Could you check a few things on this model? Use its own coordinates, in mm. A direction names the side the tool comes from. Round coordinates to 2 decimals unless told otherwise and drop trailing zeros. Loops run counter-clockwise (first coordinate to the right, second up) from the corner with the lowest first, then second, coordinate; pieces in that order, holes last. Notation, with made-up numbers: M 50.25,48 L 102.25,48 A21 ccw 102.25,66 Z; hole C 47.25,84 d10. An arc over 180 degrees is marked long. Answer in a Markdown table with one row per item.
```python
from build123d import *

# Parameters (mm, degrees)
F1_DEPTH = 25.4


with BuildPart() as f1:
    # F0 (on Front) → F1 (new body)
    with BuildSketch(Plane.XZ):
        Polygon((-82.899797516, 27.2726975213), (-82.899797516, 0.8882751458), (-18.3799119938, 0.8882751458), (-18.3799119938, 24.1686472685), align=None)
        with BuildLine():
            Line((-18.3799119938, 24.1686472685), (-18.3799119938, 0.8882751458))
            Line((-18.3799119938, 0.8882751458), (15.3484408136, 18.3339759221))
            ThreePointArc((15.3484408136, 18.3339759221), (14.2888164515, 21.1662000872), (13.9288047385, 24.1686472685))
            Line((13.9288047385, 24.1686472685), (-18.3799119938, 24.1686472685))
        make_face()
        with BuildLine():
            Line((26.6288047385, 24.1686472685), (15.3484408136, 18.3339759221))
            ThreePointArc((15.3484408136, 18.3339759221), (29.6312519198, 11.8286589814), (39.3288047385, 24.1686472685))
            ThreePointArc((39.3288047385, 24.1686472685), (26.6288047385, 36.8686472685), (13.9288047385, 24.1686472685))
            Line((13.9288047385, 24.1686472685), (26.6288047385, 24.1686472685))
        make_face()
        with BuildLine():
            ThreePointArc((13.9288047385, 24.1686472685), (14.2888164515, 21.1662000872), (15.3484408136, 18.3339759221))
            Line((15.3484408136, 18.3339759221), (26.6288047385, 24.1686472685))
            Line((26.6288047385, 24.1686472685), (13.9288047385, 24.1686472685))
        make_face()
    extrude(amount=F1_DEPTH)


solid = f1.part
```
1) I want a section at C-C, the plane x = -66.5. Please give me the cut outline in (y, z).
Computed:
| item | result |
|---|---|
| outline | M -25.4,0.89 L 0,0.89 L 0,26.48 L -25.4,26.48 Z |
2) I need wall thicknesses on line 1 (X direction, y = -6.25, z = 14); line 2 (X direction, y = -8.5, z = 3); line 3 (Z direction, x = 13, y = -19). Which ranges of each line are inside material? Lowest first, please.
Computed:
| item | result |
|---|---|
| line 1 | x = -82.9 to 6.97, 19.02 to 34.24 |
| line 2 | x = -82.9 to -14.3 |
| line 3 | z = 17.12 to 24.17 |
3) I want a section at B-B, the plane y = -20.25. Please give me the cut outline in (x, z), plus the area to 3 significant figures.
Computed:
| item | result |
|---|---|
| outline | M -82.9,0.89 L -18.38,0.89 L 15.35,18.33 A12.7 ccw long 13.93,24.17 L -18.38,24.17 L -82.9,27.27 Z |
| area | 2,590 mm² |
4) Will these pins go through, and if not, where does the flat tip stop? P1, Ø12, axis at y = -18.5, z = 4.5, coming from the +X side; P2, Ø7.5, axis at x = 1.5, y = -17.5, coming from the +Z side; P3, Ø6, axis at y = -21, z = 27, coming from the +X side; P4, Ø1, axis at y = -10.5, z = 30.5, coming from the -X side.
Computed:
| item | result |
|---|---|
| P1 | stops at x = 0.2 |
| P2 | stops at z = 24.17 |
| P3 | stops at x = 39.33 |
| P4 | stops at x = 15.35 |
5) Which directions (+Z, -Z, +X, -X, +Y, -Y) give clear straight access to the entire face, cutting with the end or side of a thin tool? Please do faces 1 (the face through (-1.75, -12.52, 9.49)), 2 (the face through (-23, -25.4, 15)), 3 (the face through (-2, -13, 24.169)).
Computed:
| item | result |
|---|---|
| face 1 | -Z, +Y, -Y |
| face 2 | +Z, -Z, +X, -X, -Y |
| face 3 | +Z, +Y, -Y |
6) I want a section at D-D, the plane z = 29. Please give me the cut outline in (x, y).
Computed:
| item | result |
|---|---|
| outline | M 14.88,-25.4 L 38.37,-25.4 L 38.37,0 L 14.88,0 Z |
7) If we mould it in two halves opening along X, with no side actions, what happens to faces 4 (the face through (-50.2, -12.5, 25.7)), 5 (the face through (-51, -13, 0.888)), 6 (the face through (-82.9, -13, 14))? For each: released by +X, released by -X, zero draft, split by the parting line, or undercut.
Computed:
| item | result |
|---|---|
| face 4 | undercut |
| face 5 | zero draft |
| face 6 | released by -X |
8) I want a section at A-A, the plane z = 16.5. Please give me the cut outline in (x, y).
Computed:
| item | result |
|---|---|
| outline | M -82.9,-25.4 L 11.8,-25.4 L 11.8,0 L -82.9,0 Z; M 16.51,-25.4 L 36.75,-25.4 L 36.75,0 L 16.51,0 Z |
